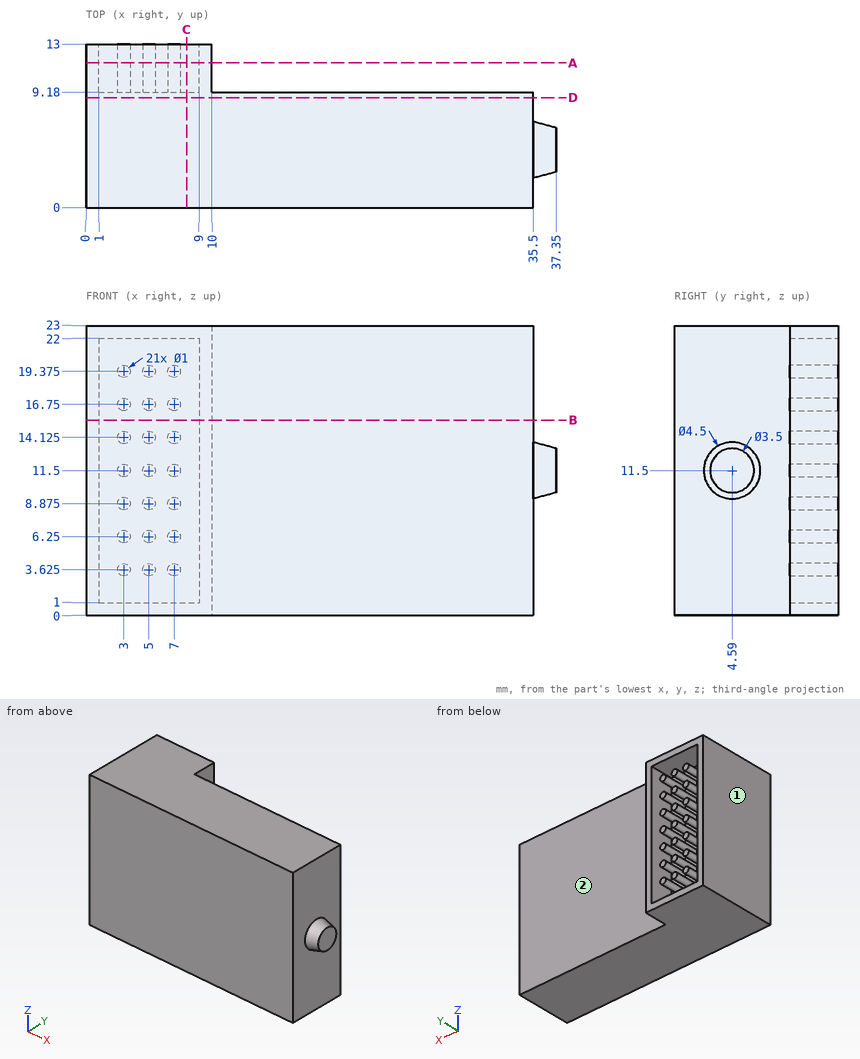
Input: dimensioned drawing with shaded views. Units: mm. Origin: part minimum x, y, z. A direction names the side the tool comes from. Coordinates: 2 decimals unless noted, no trailing zeros. Order: outer loops, then holes, each group sorted by start corner. A loop starts at its lowest first (then second) coordinate and runs counter-clockwise, first axis right, second up.
(1) First-contact query: pin 1 (12 mm diameter, centred on x = 29.5, z = 3.5, fed in from +Y); pin 2 (4 mm diameter, centred on y = 10.5, z = 8, fed in from -X); pin 3 (3 mm diameter, centred on y = 10.5, z = 13.5, fed in from +X); pin 4 (1.1 mm diameter, centred on y = 11.5, z = 13.5, fed in from +X). Flat tips, straight axial feed; report the tip coordinate or a pass-through.
(2) Section query C-C (x = 8). Return the cut outline in (y, z), plus the area to 3 significant figures.
(3) Access query for the marked faces 1 and 2. Directions: +Z, -Z, +X, -X, +Y, -Y. A direction counts if a zero-diameter tool reaches every point of the face in a straight line with its end or side. Return the directions, or none.
(4) Material intervals for probe 1 along X at (y, z) = (9.5, 13); probe 2 along Z at (x, y) = (4, 11.25); probe 3 along X at (y, z) = (3.5, 14.5), sorted ascending.
(5) Section query A-A (y = 11.5). State how many separate pieces and enclosed holes the cut face has, plus the area to 3 significant figures.
(6) Section query D-D (y = 8.75). Return the cut outline in (x, z).
(7) Section query B-B (z = 15.5). Return the cut outline in (x, y), plus the area to 3 significant figures.
Solution:
1. pin 1: stops at y = 9.18
1. pin 2: stops at x = 0
1. pin 3: stops at x = 35.5
1. pin 4: stops at x = 10
2. outline: (0, 0) - (13, 0) - (13, 1) - (9.18, 1) - (9.18, 22) - (13, 22) - (13, 23) - (0, 23) - close
2. area: 219 mm2
3. face 1: +Z, -Z, -X, +Y, -Y
3. face 2: +Z, -Z, +X, +Y
4. probe 1: x = 0 to 1, 9 to 10
4. probe 2: z = 0 to 1, 22 to 23
4. probe 3: x = 0 to 35.5
5. separate pieces: 22
5. enclosed holes: 1
5. area: 78.5 mm2
6. outline: (0, 0) - (35.5, 0) - (35.5, 23) - (0, 23) - close
7. outline: (0, 0) - (35.5, 0) - (35.5, 9.18) - (10, 9.18) - (10, 13) - (9, 13) - (9, 9.18) - (1, 9.18) - (1, 13) - (0, 13) - close
7. area: 334 mm2
